Source: three-view drawing plus pictorial views. Frame: mm from the lowest corner of the part. A direction names the side the tool comes from. Coordinates: 2 decimals unless noted, no trailing zeros. Write each loop counter-clockwise with the first axis right and the second up, starting at its lowest first coordinate (ties: lowest second). Pieces come first, ordered by that corner, then holes. Notation, with made-up numbers: (-5, -9.5) - (26, -9.5) arc R23 cw to (26, 8.5) - close; hole circle Ø9 at (-26.5, 72). An arc over 180 degrees is marked (long way). Answer as a JSON object with one key per item and string values. Group by question number.
Item 1: Section C-C on z = 17.25. Return loops of the section in (x, y) (1 decimal).
Item 2: Line query: line 1 along X through (y, z) = (2.5, 17.5) (1 decimal); line 2 along Z through (x, y) = (6.5, 2.15). Output: solid intervals per line, ascending. Write a range as from..to.
Item 3: First-contact query: pin 1 Ø1.6 at (y, z) = (1.5, 2.5) entering from +X; pin 2 Ø1.6 at (y, z) = (1.5, 16) entering from -X (1 decimal); pin 3 Ø1.6 at (x, y) = (2, 1.5) entering from +Z. Flat tips, straight axial feed; report the tip coordinate or a pass-through.
Item 4: Set-up query: the marked faces 1, 2, 3, 4 and 5. Return all of +Z, -Z, +X, -X, +Y, -Y with unobstructed straight access to the full face (end or side cutting, diameter ignored); none if empty.
Item 5: Section B-B on x = 6. Return loops of the section in (y, z) (1 decimal).
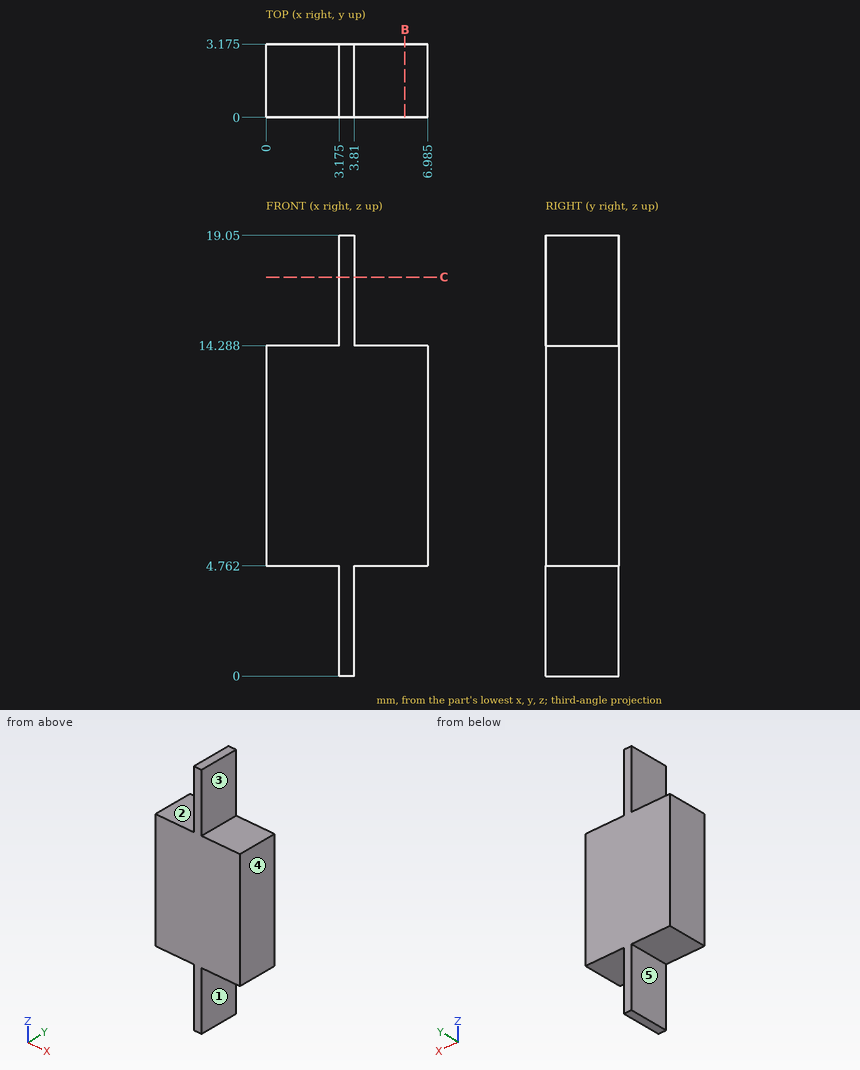
Checks:
{
 "1": {"outline": "(3.2, 0) - (3.8, 0) - (3.8, 3.2) - (3.2, 3.2) - close"},
 "2": {"line 1": "3.2..3.8", "line 2": "4.76..14.29"},
 "3": {"pin 1": "x = 3.81", "pin 2": "x = 3.2", "pin 3": "z = 14.29"},
 "4": {"face 1": "-Z, +X, +Y, -Y", "face 2": "+Z, -X, +Y, -Y", "face 3": "+Z, +X, +Y, -Y", "face 4": "+Z, -Z, +X, +Y, -Y", "face 5": "-Z, -X, +Y, -Y"},
 "5": {"outline": "(0, 4.8) - (3.2, 4.8) - (3.2, 14.3) - (0, 14.3) - close"}
}
